Could you check a few things on this model? Use its own coordinates, in mm. Face numbers are marked on the shaded views. A direction names the side the tool comes from. Give positions to 0.01 mm unless a question says otherwise; leave off trailing zeros. Write each loop counter-clockwise with the first axis right and the second up, starting at its lowest first coordinate (ties: lowest second). Pieces come first, ordered by that corner, then holes. Notation, with made-up numbers: (33.25, -18) - (82.25, -18) arc R22 ccw to (82.25, -10) - close; hole circle Ø9 at (43.5, 52). An arc over 180 degrees is marked (long way). Use one line per item in the form item = value.
```python
from build123d import *

# Parameters (mm, degrees)
F0_W     = 177.8
F0_H     = 63.5
F1_DEPTH = 6.35
F2_W     = 127
F2_H     = 31.75
F3_DEPTH = 254
F4_R     = 30
F5_DEPTH = 5


with BuildPart() as f1:
    # F0 (on Front) → F1 (new body)
    with BuildSketch(Plane.XZ):
        Rectangle(F0_W, F0_H)
    extrude(amount=F1_DEPTH)

    # F2 (on face) → F3 (join)
    with BuildSketch(Plane(origin=(0, 0, 0), x_dir=(-1, 0, 0), z_dir=(0, 1, 0))):
        with Locations((0, -15.875)):
            Rectangle(F2_W, F2_H)
    extrude(amount=F3_DEPTH)

    # F4 (on face) → F5 (cut)
    with BuildSketch(Plane.XY):
        with Locations((-18.2372, 169.2656)):
            Circle(F4_R)
    extrude(amount=-F5_DEPTH, mode=Mode.SUBTRACT)


solid = f1.part
```
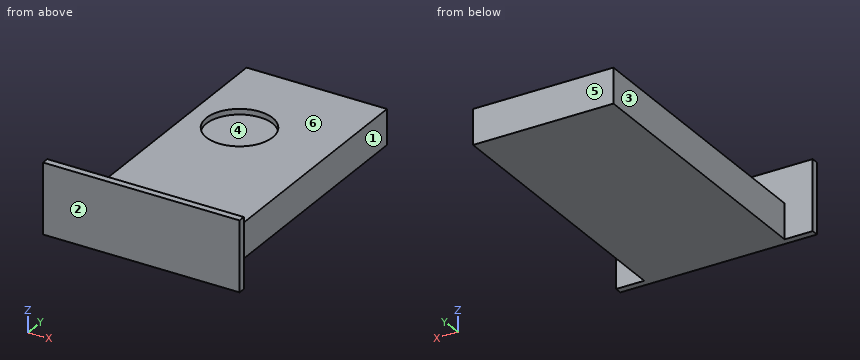
1. Which directions (+Z, -Z, +X, -X, +Y, -Y) give clear straight access to the entire face, cutting with the end or side of a thin tool? Please do the marked faces 5 and 6.
Response values:
face_5 = +Z, -Z, +X, -X, +Y
face_6 = +Z, +X, -X, +Y
2. Imagine slicing it at A-A, the plane z = -23.5. List the corners of the cut face in (x, y) for me, and give its area (3 significant figures).
Response values:
outline = (-88.9, -6.35) - (88.9, -6.35) - (88.9, 0) - (63.5, 0) - (63.5, 254) - (-63.5, 254) - (-63.5, 0) - (-88.9, 0) - close
area = 33,400 mm²
3. Imagine slicing it at D-D, the plane x = -21.5. List the corners of the cut face in (y, z) for me.
Response values:
outline = (-6.35, -31.75) - (254, -31.75) - (254, 0) - (199.09, 0) - (199.09, -5) - (139.44, -5) - (139.44, 0) - (0, 0) - (0, 31.75) - (-6.35, 31.75) - close
4. For pin 1 (9.5 mm diameter, centred on y = 177, z = -19, fed in from -X); pin 2 (5 mm diameter, centred on x = -8, z = 7.5, fed in from +Y); pin 3 (9.5 mm diameter, centred on y = 77, z = -13, fed in from +X), each with a flat end and sliding along its axis, tell me the tip position at first contact or that it passes through.
Response values:
pin_1 = -63.5
pin_2 = 0
pin_3 = 63.5
5. If we mould it in two halves opening along X, with no side actions, what happens to the marked faces 1, 2, 3 and 4? For each: pulls with the +X half, pulls with the -X half, needs draft (parallel to the pull), parting line crosses it, or undercut.
Response values:
face_1 = pulls with the +X half
face_2 = needs draft
face_3 = pulls with the -X half
face_4 = undercut
6. If I drill on line 1 (X direction, y = 98, z = -14.5); line 2 (Y direction, x = 21, z = 28); line 3 (Z direction, x = 1.5, y = 204), over which ranges is the centre line in solid material (lowest first)? Write a range as from..to.
Response values:
line_1 = -63.5..63.5
line_2 = -6.35..0
line_3 = -31.75..0
7. Imagine slicing it at B-B, the plane x = 5. List the corners of the cut face in (y, z) for me.
Response values:
outline = (-6.35, -31.75) - (254, -31.75) - (254, 0) - (188.24, 0) - (188.24, -5) - (150.29, -5) - (150.29, 0) - (0, 0) - (0, 31.75) - (-6.35, 31.75) - close
8. Imagine slicing it at C-C, the plane y = 177.5. List the corners of the cut face in (x, z) for me, and give its area (3 significant figures).
Response values:
outline = (-63.5, -31.75) - (63.5, -31.75) - (63.5, 0) - (10.61, 0) - (10.61, -5) - (-47.08, -5) - (-47.08, 0) - (-63.5, 0) - close
area = 3,740 mm²
